Design review of the part built by this model. Coordinates are the model's own, in mm. A direction names the side the tool comes from. Give positions to 0.01 mm unless a question says otherwise; leave off trailing zeros. Order: outer loops, then holes, each group sorted by start corner. A loop starts at its lowest first (then second) coordinate and runs counter-clockwise, first axis right, second up.
```python
from build123d import *

# Parameters (mm, degrees)
F0_W = 7.45
F0_H = 9.95


# Not quite as in the source:
# - a feature names something its author has since deleted; it is built from what else it names


with BuildPart() as f1:
    # F0 (on Front) → F1 (revolve)
    with BuildSketch(Plane.XZ):
        Polygon((0, 2.35), (0, 0), (17, 0), (17, 15.7), (9.55, 15.7), (0, 15.7), (0, 13.35), (3, 13.35), (3, 2.35), align=None)
        with Locations((13.275, 20.675)):
            Rectangle(F0_W, F0_H)
    revolve(axis=Axis((27, 0, 7.85), (0, 0, 1)))


solid = f1.part
```
1. Draft analysis for pull direction Z (two halves, no side actions). For faces 4 (the face through (15, 0, 0)), 5 (the face through (51.1, 1.9, 13.35)), 6 (the face through (2.06, 10.34, 14.51)), 7 (the face through (50.977, -1.055, 7.773)), state which applies: pulls with the +Z half, pulls with the -Z half, needs draft (parallel to the pull), parting line crosses it, or undercut.
Recorded:
face 4: pulls with the -Z half
face 5: undercut
face 6: needs draft
face 7: undercut
2. Take a section at C-C (z = 22.5). State the section outline as (x, y) points.
Recorded:
outline: circle Ø34.9 at (27, 0); hole circle Ø20 at (27, 0)
3. Take a section at D-D (x = 11). State the section outline as (y, z) points.
Recorded:
outline: (-21.75, 0) - (21.75, 0) - (21.75, 2.35) - (17.89, 2.35) - (17.89, 13.35) - (21.75, 13.35) - (21.75, 15.7) - (6.96, 15.7) - (6.96, 25.65) - (-6.96, 25.65) - (-6.96, 15.7) - (-21.75, 15.7) - (-21.75, 13.35) - (-17.89, 13.35) - (-17.89, 2.35) - (-21.75, 2.35) - close
4. Take a section at A-A (x = 27). State the section outline as (y, z) points.
Recorded:
outline: (-27, 0) - (-10, 0) - (-10, 25.65) - (-17.45, 25.65) - (-17.45, 15.7) - (-27, 15.7) - (-27, 13.35) - (-24, 13.35) - (-24, 2.35) - (-27, 2.35) - close; (10, 0) - (27, 0) - (27, 2.35) - (24, 2.35) - (24, 13.35) - (27, 13.35) - (27, 15.7) - (17.45, 15.7) - (17.45, 25.65) - (10, 25.65) - close
5. Machinability: for faces 1 (the face through (2.9, 1.9, 2.35)), 2 (the face through (2.06, 10.34, 1.16)), 3 (the face through (27, 18, 15.7)), which of the approach directions +Z, -Z, +X, -X, +Y, -Y give a long, thin tool a straight path to every point of the face, cutting with its end or side? Answer none if there is none.
Recorded:
face 1: none
face 2: +Z, -Z
face 3: +Z
6. For pin 1 (4 mm diameter, centred on y = 2, z = 23, fed in from -X); pin 2 (3 mm diameter, centred on y = -7.5, z = 5.5, fed in from +X); pin 3 (2 mm diameter, centred on y = -9, z = 12, fed in from +X), all flat-tipped, find the tip position at first contact; note any pin that passes through.
Recorded:
pin 1: stops at x = 9.55
pin 2: stops at x = 50.24
pin 3: stops at x = 49.63
7. For line 1 along X through (y, z) = (0, 10); line 2 along Z through (x, y) = (42.5, -9); line 3 along Y through (x, z) = (27, 18.75), list the stretches that pass through material, from the lowest coordinate up.
Recorded:
line 1: x = 3 to 17, 37 to 51
line 2: z = 0 to 15.7
line 3: y = -17.45 to -10, 10 to 17.45
8. Take a section at B-B (y = 0). State the section outline as (x, z) points, then the cut area to 3 significant figures.
Recorded:
outline: (0, 0) - (17, 0) - (17, 25.65) - (9.55, 25.65) - (9.55, 15.7) - (0, 15.7) - (0, 13.35) - (3, 13.35) - (3, 2.35) - (0, 2.35) - close; (37, 0) - (54, 0) - (54, 2.35) - (51, 2.35) - (51, 13.35) - (54, 13.35) - (54, 15.7) - (44.45, 15.7) - (44.45, 25.65) - (37, 25.65) - close
area: 616 mm2
